```python
from build123d import *

# Parameters (mm, degrees)
BOSS_EXTRUDE1_DEPTH = 30
CUT_EXTRUDE1_DEPTH  = 121
BOSS_EXTRUDE2_DEPTH = 10
CUT_EXTRUDE2_DEPTH  = 21
CUT_EXTRUDE3_DEPTH  = 21


with BuildPart() as part:
    # Sketch1 → Boss-Extrude1 (new body, symmetric)
    with BuildSketch(Plane.XY):
        Polygon((-60, 0), (60, 0), (60, 50), (50, 50), (50, 10), (-50, 10), (-50, 50), (-60, 50), align=None)
    extrude(amount=BOSS_EXTRUDE1_DEPTH, both=True)

    # Sketch2 → Cut-Extrude1 (cut, through all)
    with BuildSketch(Plane(origin=(60, 0, 0), x_dir=(0, 0, -1), z_dir=(1, 0, 0))):
        with BuildLine():
            Line((-7.5, 35), (-7.5, 50))
            Line((-7.5, 50), (7.5, 50))
            Line((7.5, 50), (7.5, 35))
            ThreePointArc((7.5, 35), (0, 27.5), (-7.5, 35))
        make_face()
    extrude(amount=-CUT_EXTRUDE1_DEPTH, mode=Mode.SUBTRACT)

    # Sketch3 → Boss-Extrude2 (add)
    with BuildSketch(Plane(origin=(0, 10, 0), x_dir=(1, 0, 0), z_dir=(0, 1, 0))):
        Polygon((0, 30), (30, 0), (0, -30), (-30, 0), align=None)
    extrude(amount=BOSS_EXTRUDE2_DEPTH)

    # Sketch4 → Cut-Extrude2 (cut, through all)
    with BuildSketch(Plane(origin=(0, 20, 0), x_dir=(1, 0, 0), z_dir=(0, 1, 0))):
        Polygon((0, 8.485281374), (8.485281374, 0), (0, -8.485281374), (-8.485281374, 0), align=None)
    extrude(amount=-CUT_EXTRUDE2_DEPTH, mode=Mode.SUBTRACT)

    # Sketch5 → Cut-Extrude3 (cut, through all)
    with BuildSketch(Plane(origin=(0, 20, 0), x_dir=(1, 0, 0), z_dir=(0, 1, 0))):
        with BuildLine():
            Line((10.757359313, 19.242640687), (19.242640687, 10.757359313))
            ThreePointArc((19.242640687, 10.757359313), (19.242640687, 19.242640687), (10.757359313, 19.242640687))
        make_face()
        with BuildLine():
            Line((19.242640687, -10.757359313), (10.757359313, -19.242640687))
            ThreePointArc((10.757359313, -19.242640687), (19.242640687, -19.242640687), (19.242640687, -10.757359313))
        make_face()
        with BuildLine():
            Line((-10.757359313, -19.242640687), (-19.242640687, -10.757359313))
            ThreePointArc((-19.242640687, -10.757359313), (-19.242640687, -19.242640687), (-10.757359313, -19.242640687))
        make_face()
        with BuildLine():
            Line((-19.242640687, 10.757359313), (-10.757359313, 19.242640687))
            ThreePointArc((-10.757359313, 19.242640687), (-19.242640687, 19.242640687), (-19.242640687, 10.757359313))
        make_face()
    extrude(amount=-CUT_EXTRUDE3_DEPTH, mode=Mode.SUBTRACT)


solid = part.part
```
Part model, mm, in its own coordinate system. A direction names the side the tool comes from. Round coordinates to 2 decimals unless told otherwise and drop trailing zeros. Loops run counter-clockwise (first coordinate to the right, second up) from the corner with the lowest first, then second, coordinate; pieces in that order, holes last.
1. Slice it at D-D (y = 42). Give the cut face in (x, z), and give its area (3 significant figures).
Solutions:
outline: (-60, -30) - (-50, -30) - (-50, -7.5) - (-60, -7.5) - close; (-60, 7.5) - (-50, 7.5) - (-50, 30) - (-60, 30) - close; (50, -30) - (60, -30) - (60, -7.5) - (50, -7.5) - close; (50, 7.5) - (60, 7.5) - (60, 30) - (50, 30) - close
area: 900 mm2
2. Drill centre lines: line 1 along X through (y, z) = (35, -13.5); line 2 along X through (y, z) = (12, 21); line 3 along Y through (x, z) = (47, -1). Where is each one in solid material? Low to high.
Solutions:
line 1: x = -60 to -50, 50 to 60
line 2: x = -60 to -50, -9 to 9, 50 to 60
line 3: y = 0 to 10
3. Two-plate mould, pull along X, no slides. Class faces 4 (the face through (60, 25, 0)), 5 (the face through (4.183, 10.14, -4.302)), 6 (the face through (55.07, 27.5, -0.16)): pulls with the +X half, pulls with the -X half, needs draft (parallel to the pull), parting line crosses it, or undercut.
Solutions:
face 4: pulls with the +X half
face 5: undercut
face 6: needs draft
4. Slice it at B-B (z = -15). Give the cut face in (x, y).
Solutions:
outline: (-60, 0) - (-21, 0) - (-21, 10) - (-50, 10) - (-50, 50) - (-60, 50) - close; (-15, 0) - (15, 0) - (15, 20) - (-15, 20) - close; (21, 0) - (60, 0) - (60, 50) - (50, 50) - (50, 10) - (21, 10) - close
5. Slice it at C-C (y = 24.5). Give the cut face in (x, z).
Solutions:
outline: (-60, -30) - (-50, -30) - (-50, 30) - (-60, 30) - close; (50, -30) - (60, -30) - (60, 30) - (50, 30) - close
6. Slice it at A-A (x = -15). Give the cut face in (y, z), and give its area (3 significant figures).
Solutions:
outline: (0, -30) - (10, -30) - (10, -21) - (0, -21) - close; (0, -15) - (20, -15) - (20, 15) - (0, 15) - close; (0, 21) - (10, 21) - (10, 30) - (0, 30) - close
area: 780 mm2
7. 3-axis set-ups, long thin cutter, end or side, ignore diameter. For faces 1 (the face through (50, 26, 0)), 2 (the face through (55, 43, -7.5)), 3 (the face through (-30.2, 10, 0.4)): which of +Z, -Z, +X, -X, +Y, -Y reach the whole face in a straight line?
Solutions:
face 1: +Z, -Z, +Y
face 2: +X, -X, +Y
face 3: +Y
